from build123d import *

# Parameters (mm, degrees)
F1_DEPTH = 10


with BuildPart() as f1:
    # F0 (on Top) → F1 (new body)
    with BuildSketch(Plane.XY):
        Polygon((22.2, 1.5), (21.4, 1.5), (21.4, 2.35), (0, 2.35), (0, 0), (0, -2.35), (21.4, -2.35), (21.4, -1.5), (22.2, -1.5), (23.05, -2.35), (23.75, -2.35), (24, -2.1), (24, 0), (24, 2.1), (23.75, 2.35), (23.05, 2.35), align=None)
    extrude(amount=-F1_DEPTH)


solid = f1.part
For this review, take the finished solid that the model builds, in its own axes (mm). A direction names the side the tool comes from. Round coordinates to 2 decimals unless told otherwise and drop trailing zeros. Loops run counter-clockwise (first coordinate to the right, second up) from the corner with the lowest first, then second, coordinate; pieces in that order, holes last. Notation, with made-up numbers: (89, 59.25) - (148, 59.25) arc R21 cw to (148, 74.25) - close; hole circle Ø1 at (6, 74.5). An arc over 180 degrees is marked (long way). One line per question, with ' | ' between items.
Q1. Take a section at A-A (y = -1.85). Give the boundary of the cut face in (x, z).
Taken from the geometry:
outline: (0, -10) - (21.4, -10) - (21.4, 0) - (0, 0) - close; (22.55, -10) - (24, -10) - (24, 0) - (22.55, 0) - close
Q2. Take a section at B-B (z = -2.5). Give the boundary of the cut face in (x, y), and give its area (3 significant figures).
Taken from the geometry:
outline: (0, -2.35) - (21.4, -2.35) - (21.4, -1.5) - (22.2, -1.5) - (23.05, -2.35) - (23.75, -2.35) - (24, -2.1) - (24, 2.1) - (23.75, 2.35) - (23.05, 2.35) - (22.2, 1.5) - (21.4, 1.5) - (21.4, 2.35) - (0, 2.35) - close | area: 111 mm²
Q3. The part is to be moulded in two halves that separate along X. For faces 4 (the flat face through (22, 1.5, -5)), 5 (the flat face through (12, 0, 0)), 6 (the flat face through (22.6, 1.9, -4.9)), 7 (the flat face through (0, 0, -5)), say which applies: released by +X, released by -X, zero draft, split by the parting line, or undercut.
Taken from the geometry:
face 4: undercut | face 5: zero draft | face 6: undercut | face 7: released by -X
Q4. For line 1 along X through (y, z) = (-1.55, -9); line 2 along X through (y, z) = (1.6, -9.25), list the stretches that pass through material, from the lowest coordinate up. Write a range as [from, to].
Taken from the geometry:
line 1: x = [0, 21.4], [22.25, 24] | line 2: x = [0, 21.4], [22.3, 24]
Q5. Tool access review of faces 1 (the flat face through (22, -1.5, -5)), 2 (the flat face through (21.4, 2, -5)), 3 (the flat face through (11, 2.35, -5)): name each direction out of +Z, -Z, +X, -X, +Y, -Y from which nothing blocks a thin tool from reaching the whole face with its end or side.
Taken from the geometry:
face 1: +Z, -Z, -Y | face 2: +Z, -Z, +Y | face 3: +Z, -Z, +X, -X, +Y
